Part model, mm, in its own coordinate system. A direction names the side the tool comes from. Round coordinates to 2 decimals unless told otherwise and drop trailing zeros. Loops run counter-clockwise (first coordinate to the right, second up) from the corner with the lowest first, then second, coordinate; pieces in that order, holes last. Notation, with made-up numbers: M 33.25,41 L 69.25,41 A30 ccw 69.25,74 Z; hole C -19.5,76.5 d1. An arc over 180 degrees is marked long. Put each result on its own line as item: value. Start each with the question number.
```python
from build123d import *

# Parameters (mm, degrees)
BOSS_EXTRUDE1_DEPTH = 19
BOSS_EXTRUDE2_DEPTH = 7
SKETCH3_R           = 1.75
CUT_EXTRUDE1_DEPTH  = 37.75
SKETCH6_R           = 4
CUT_EXTRUDE4_DEPTH  = 4
SKETCH7_R           = 1.625
CUT_EXTRUDE5_DEPTH  = 20
FILLET1_R           = 2
SKETCH8_R           = 1.75
CUT_EXTRUDE6_DEPTH  = 10
SKETCH9_R           = 4
CUT_EXTRUDE7_DEPTH  = 4


with BuildPart() as part:
    # Sketch1 → Boss-Extrude1 (new body)
    with BuildSketch(Plane.XY):
        Polygon((0, 0), (20, 0), (20, 43.25), (-16.75, 43.25), (-16.75, 36), (0, 36), align=None)
    extrude(amount=BOSS_EXTRUDE1_DEPTH)

    # Sketch2 → Boss-Extrude2 (add)
    with BuildSketch(Plane(origin=(0, 0, 0), x_dir=(-1, 0, 0), z_dir=(0, 0, -1))):
        with BuildLine():
            Line((-20, 36), (16.75, 36))
            Line((16.75, 36), (16.75, 68))
            Line((16.75, 68), (7.25, 77.5))
            Line((7.25, 77.5), (4.5, 77.5))
            Line((4.5, 77.5), (2, 75))
            Line((2, 75), (2, 59.75))
            ThreePointArc((2, 59.75), (-7.896468276, 45.089682755), (-20.5, 57.5))
            Line((-20.5, 57.5), (-25, 57.5))
            Line((-25, 57.5), (-30, 52.5))
            Line((-30, 52.5), (-30, 37.5))
            Line((-30, 37.5), (-28.5, 36))
            Line((-28.5, 36), (-20, 36))
        make_face()
    extrude(amount=-BOSS_EXTRUDE2_DEPTH)

    # Sketch3 → Cut-Extrude1 (cut, through all)
    with BuildSketch(Plane(origin=(20, 0, 0), x_dir=(0, 0, -1), z_dir=(1, 0, 0))):
        with Locations((-8.25, 26.25)):
            Circle(SKETCH3_R)
        with Locations((-8.25, 6.25)):
            Circle(SKETCH3_R)
    extrude(amount=-CUT_EXTRUDE1_DEPTH, mode=Mode.SUBTRACT)

    # Sketch6 → Cut-Extrude4 (cut)
    with BuildSketch(Plane(origin=(20, 0, 0), x_dir=(0, 0, -1), z_dir=(1, 0, 0))):
        with Locations((-8.25, 26.25)):
            Circle(SKETCH6_R)
        with Locations((-8.25, 6.25)):
            Circle(SKETCH6_R)
    extrude(amount=-CUT_EXTRUDE4_DEPTH, mode=Mode.SUBTRACT)

    # Sketch7 → Cut-Extrude5 (cut, through all)
    with BuildSketch(Plane(origin=(0, 0, 0), x_dir=(-1, 0, 0), z_dir=(0, 0, -1))):
        with Locations((6.5, 72.5)):
            Circle(SKETCH7_R)
        with Locations((-24.5, 41.5)):
            Circle(SKETCH7_R)
    extrude(amount=-CUT_EXTRUDE5_DEPTH, mode=Mode.SUBTRACT)

    # Fillet1
    fillet1_edges = [part.edges().sort_by_distance(p)[0] for p in [
        (20, 43.25, 13),
        (20, 0, 9.5),
        (30, 52.5, 3.5),
    ]]
    fillet(fillet1_edges, radius=FILLET1_R)

    # Sketch8 → Cut-Extrude6 (cut)
    with BuildSketch(Plane.XZ.offset(-36)):
        with Locations((-10, 14)):
            Circle(SKETCH8_R)
    extrude(amount=-CUT_EXTRUDE6_DEPTH, mode=Mode.SUBTRACT)

    # Sketch9 → Cut-Extrude7 (cut)
    with BuildSketch(Plane(origin=(0, 43.25, 0), x_dir=(1, 0, 0), z_dir=(0, 1, 0))):
        with Locations((-10, -14)):
            Circle(SKETCH9_R)
    extrude(amount=-CUT_EXTRUDE7_DEPTH, mode=Mode.SUBTRACT)


solid = part.part
```
1. Cut at D-D, the plane z = 13.25. Give the cut face in (x, y), and give its area (3 significant figures).
2. Mould opens along Z. For faces 5 (the flat face through (16, 4.5, 7.4)), 6 (the flat face through (24, 36, 3)), 7 (the cylindrical face through (18.028, 3.816, 11.424)), 8 (the flat face through (5, 27, 19)) say: released by +Z, released by -Z, zero draft, split by the parting line, or undercut.
3. Cut at B-B, the plane y = 26.25. Give the cut face in (x, z), and give its area (3 significant figures).
4. Cut at C-C, the plane z = 8.25. Give the cut face in (x, y), and give its area (3 significant figures).
5. Drop flat-ended pins along their axis: pin 1 (1 mm diameter, centred on x = -8, y = 45.5, fed in from +Z); pin 2 (2 mm diameter, centred on x = 23.5, z = 3.5, fed in from +Y); pin 3 (3 mm diameter, centred on y = 6.25, z = 8.25, fed in from +X); pin 4 (5 mm diameter, centred on x = 14.5, z = 10.5, fed in from +Y). Give the stop position or say it passes through.
6. Which spindle directions (+Z, -Z, +X, -X, +Y, -Y) get a long thin tool onto all of the face, cutting with end or side? Do faces 1 (the flat face through (-2, 67, 3)), 2 (the flat face through (-8, 36, 9)), 3 (the flat face through (-9, 39.25, 16)), 4 (the cylindrical face through (19.43, 42.65, 13.08)). Say none if no direction does.
7. Cut at A-A, the plane x = -10. Give the cut face in (y, z), and give its area (3 significant figures).
8. Wall check: L1, parallel to Y at x = 10.75, z = 8.25; L2, parallel to Y at x = 17.2, z = 8.25; L3, parallel to Z at x = 17, y = 26. Give the ranges that are in metal, low to high.
Results list:
1. outline: M -16.75,36 L -11.58,36 L -11.58,39.25 L -13.93,39.25 L -13.93,43.25 L -16.75,43.25 Z; M -8.42,36 L 0,36 L 0,0 L 18,0 A2 ccw 20,2 L 20,41.25 A2 ccw 18,43.25 L -6.07,43.25 L -6.07,39.25 L -8.42,39.25 Z
1. area: 943 mm^2
2. face 5: undercut
2. face 6: zero draft
2. face 7: undercut
2. face 8: released by +Z
3. outline: M 0,0 L 20,0 L 20,4.25 L 16,4.25 L 16,6.5 L 0,6.5 Z; M 0,10 L 16,10 L 16,12.25 L 20,12.25 L 20,19 L 0,19 Z
3. area: 292 mm^2
4. outline: M -16.75,36 L 0,36 L 0,28 L 16,28 L 16,30.25 L 20,30.25 L 20,41.25 A2 ccw 18,43.25 L -16.75,43.25 Z; M 0,0 L 18,0 A2 ccw 20,2 L 20,2.25 L 16,2.25 L 16,4.5 L 0,4.5 Z; M 0,8 L 16,8 L 16,10.25 L 20,10.25 L 20,22.25 L 16,22.25 L 16,24.5 L 0,24.5 Z
4. area: 809 mm^2
5. pin 1: stops at z = 7
5. pin 2: stops at y = 57.5
5. pin 3: passes through
5. pin 4: stops at y = 43.25
6. face 1: +Z, -Z, +X, +Y
6. face 2: +Z, -Z, -X, -Y
6. face 3: +Y
6. face 4: +Z, +X, +Y
7. outline: M 36,0 L 74.75,0 L 74.75,7 L 43.25,7 L 43.25,10 L 39.25,10 L 39.25,12.25 L 36,12.25 Z; M 36,15.75 L 39.25,15.75 L 39.25,18 L 43.25,18 L 43.25,19 L 36,19 Z
7. area: 315 mm^2
8. L1: y = 0 to 4.5, 8 to 24.5, 28 to 43.25
8. L2: y = 0 to 2.25, 10.25 to 22.25, 30.25 to 43.25
8. L3: z = 0 to 4.26, 12.24 to 19
